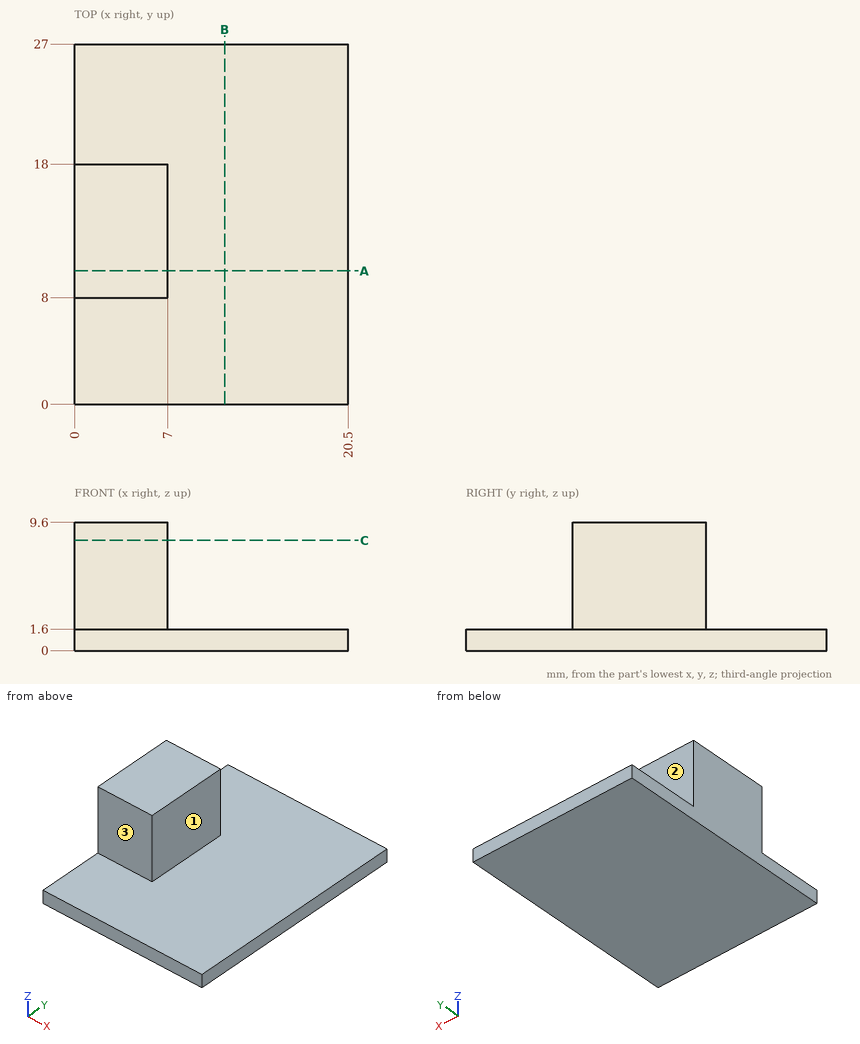
Answer from the drawing. Dimensions are ordinates in mm from the lowest x, y and z of the part. A direction names the side the tool comes from. Coordinates: 2 decimals unless noted, no trailing zeros. Order: outer loops, then holes, each group sorted by start corner. A loop starts at its lowest first (then second) coordinate and runs counter-clockwise, first axis right, second up. Notation, with made-up numbers: (64, -5.75) - (76, -5.75) arc R17 cw to (76, 12.25) - close; hole circle Ø6 at (-31, 7.5). An arc over 180 degrees is marked (long way). Answer as a JSON object with one key per item and string values. Group by question number.
Item 1: Section A-A (y = 10) is taken. Give the vertices of the cut face in (x, z).
Item 2: Consider probe 1 along Z at (x, y) = (12.5, 24); probe 2 along X at (y, z) = (13, 7); probe 3 along Y at (x, z) = (1.5, 5.75). Determine where each line is inside the solid, lowest interval first. Write a range as from..to.
Item 3: Section B-B (x = 11.25) is taken. Give the vertices of the cut face in (y, z).
Item 4: A tool of negligible diameter and unlimited length cuts with its end or side. For the marked faces 1, 2 and 3, from which of +Z, -Z, +X, -X, +Y, -Y can it reach the whole face along a straight path? Write none if from no direction.
Item 5: Flat-ended cylindrical pins translate along their axes: P1, Ø6, axis at x = 15, y = 7.5, coming from the +Z side; P2, Ø5.5, axis at x = 5, z = 6, coming from the +Y side; P3, Ø2, axis at y = 8, z = 8, coming from the +X side. Find the tip coordinate at first contact, or state that the pin passes through.
Item 6: Section C-C (z = 8.25) is taken. Give the vertices of the cut face in (x, y), plus the area to 3 significant figures.
Results are:
{
 "1": {"outline": "(0, 0) - (20.5, 0) - (20.5, 1.6) - (7, 1.6) - (7, 9.6) - (0, 9.6) - close"},
 "2": {"probe 1": "z = 0..1.6", "probe 2": "x = 0..7", "probe 3": "y = 8..18"},
 "3": {"outline": "(0, 0) - (27, 0) - (27, 1.6) - (0, 1.6) - close"},
 "4": {"face 1": "+Z, +X, +Y, -Y", "face 2": "+Z, +X, -X, +Y", "face 3": "+Z, +X, -X, -Y"},
 "5": {"P1": "stops at z = 1.6", "P2": "stops at y = 18", "P3": "stops at x = 7"},
 "6": {"outline": "(0, 8) - (7, 8) - (7, 18) - (0, 18) - close", "area": "70.0 mm^2"}
}
